```python
from build123d import *

# Parameters (mm, degrees)
SKETCH_1_W                     = 305.5
SKETCH_1_H                     = 1221.15
EXTRUDE_1_DEPTH                = 4.75
CUT_EXTRUDE_2_DEPTH            = 4.75
SPLIT_BODIES_1_SURFACE_1_BACK  = 1259.793
SPLIT_BODIES_1_SURFACE_1_DEPTH = 2519.586


with BuildPart() as part:
    # 草圖1 → 填料-伸長1 (new body)
    with BuildSketch(Plane.XY):
        Rectangle(SKETCH_1_W, SKETCH_1_H)
    extrude(amount=EXTRUDE_1_DEPTH)

    # 草圖2 → 除料-伸長2 (cut)
    with BuildSketch(Plane.XY.offset(4.75)):
        Polygon((100.025, 354.412698413), (100.025, 304.423280423), (-83.25542328, 382.984126984), (-99.975, 390.137566138), (-99.975, 440.126984127), (83.30542328, 361.566137566), align=None)
        Polygon((57.189021164, 380.021164021), (57.189021164, 440.126984127), (100.025, 440.126984127), (100.025, 361.566137566), align=None)
        Polygon((50.035582011, 106.53968254), (57.189021164, 106.53968254), (57.189021164, 120.846560847), (100.025, 120.846560847), (100.025, 84.994708995), (71.453571429, 56.55026455), (50.035582011, 56.55026455), align=None)
        Polygon((-71.403571429, 56.55026455), (-99.975, 84.994708995), (-99.975, 120.846560847), (-57.096693122, 120.846560847), (-57.096693122, 106.53968254), (-21.414153439, 106.53968254), (-21.414153439, 120.846560847), (21.464153439, 120.846560847), (21.464153439, 85.121693122), (-7.107275132, 56.55026455), align=None)
        Polygon((-21.414153439, 142.264550265), (-57.096693122, 142.264550265), (-57.096693122, 127.830687831), (-99.975, 128), (-99.975, 163.682539683), (-71.403571429, 192.423280423), (71.453571429, 192.253968254), (100.025, 163.682539683), (100.025, 127.830687831), (57.189021164, 127.830687831), (57.189021164, 142.264550265), (21.464153439, 142.264550265), (21.464153439, 128), (-21.414153439, 128), align=None)
        Polygon((21.591137566, -141.164021164), (57.189021164, -141.164021164), (57.189021164, -127.026455026), (100.025, -127.026455026), (100.025, -162.878306878), (71.453571429, -191.322751323), (7.157275132, -191.322751323), (0.046164021, -184.042328042), (-6.980291005, -191.44973545), (-71.276587302, -191.44973545), (-99.848015873, -163.047619048), (-99.975, -127.026455026), (-57.096693122, -127.026455026), (-56.969708995, -141.333333333), (-21.24484127, -141.333333333), (-21.414153439, -127.026455026), (21.29484127, -126.899470899), (21.29484127, -127.153439153), (21.591137566, -127.153439153), align=None)
        Polygon((50.035582011, -55.44973545), (71.453571429, -55.44973545), (100.025, -84.19047619), (100.025, -120.042328042), (57.189021164, -120.042328042), (57.189021164, -105.608465608), (50.035582011, -105.608465608), align=None)
        Polygon((-49.985582011, -105.608465608), (-57.096693122, -105.608465608), (-57.096693122, -120.042328042), (-99.975, -119.873015873), (-99.975, -84.19047619), (-71.403571429, -55.44973545), (-49.985582011, -55.44973545), align=None)
        Polygon((50.035582011, -389.206349206), (57.189021164, -389.206349206), (57.189021164, -374.899470899), (100.025, -374.899470899), (100.025, -410.751322751), (71.453571429, -439.195767196), (50.035582011, -439.195767196), align=None)
        Polygon((-71.403571429, -439.195767196), (-99.975, -410.751322751), (-99.975, -374.899470899), (-57.096693122, -374.899470899), (-57.096693122, -389.206349206), (-21.414153439, -389.206349206), (-21.414153439, -374.899470899), (21.464153439, -374.899470899), (21.464153439, -410.624338624), (-7.107275132, -439.195767196), align=None)
        Polygon((-21.414153439, -353.481481481), (-57.096693122, -353.481481481), (-57.096693122, -367.915343915), (-99.975, -367.746031746), (-99.975, -332.063492063), (-71.403571429, -303.322751323), (71.453571429, -303.492063492), (100.025, -332.063492063), (100.025, -367.915343915), (57.189021164, -367.915343915), (57.189021164, -353.481481481), (21.464153439, -353.481481481), (21.464153439, -367.746031746), (-21.414153439, -367.746031746), align=None)
    extrude(amount=-CUT_EXTRUDE_2_DEPTH, mode=Mode.SUBTRACT)

    # Split Bodies 1: cut with a surface, the side it looks to stays
    # Split Bodies 1 surface: a surface, the sketch's curves swept straight by 2519.586 mm
    with BuildLine(Plane.XY.offset(4.75).offset(-SPLIT_BODIES_1_SURFACE_1_BACK), mode=Mode.PRIVATE) as split_bodies_1_surface_1_path:
        Line((-152.75, 205.025), (152.75, 205.025))
    split_bodies_1_surface_1 = Shell.extrude(split_bodies_1_surface_1_path.wire(), (0 * SPLIT_BODIES_1_SURFACE_1_DEPTH, 0 * SPLIT_BODIES_1_SURFACE_1_DEPTH, 1 * SPLIT_BODIES_1_SURFACE_1_DEPTH))
    split(bisect_by=split_bodies_1_surface_1, keep=Keep.TOP)


solid = part.part
```
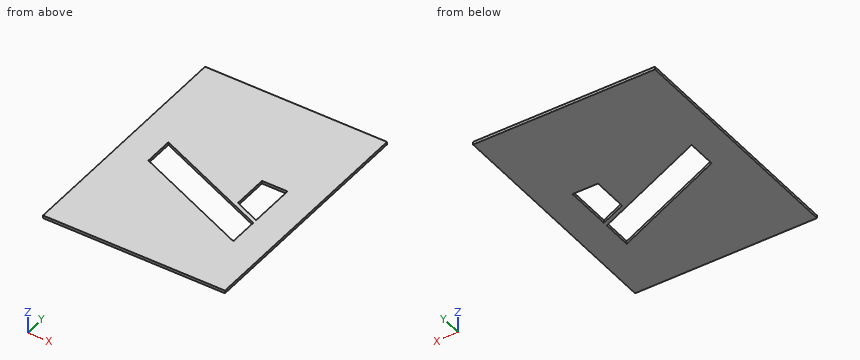
Design review of the part built by this model. Coordinates are the model's own, in mm. Round coordinates to 2 decimals unless told otherwise and drop trailing zeros. Write each loop counter-clockwise with the first axis right and the second up, starting at its lowest first coordinate (ties: lowest second). Pieces come first, ordered by that corner, then holes. Notation, with made-up numbers: (18, 0.5) -> (46, 0.5) arc R20 ccw to (46, 20.5) -> close; hole circle Ø4 at (57.25, 50.25). An arc over 180 degrees is marked (long way). Answer in a Markdown table with one row per item.
Q1. Take a section at B-B, the plane x = 33. State the section outline as (y, z) points (3 decimals), then the cut area to 3 significant figures.
The answers:
| item | result |
|---|---|
| outline | (205.025, 0) -> (333.153, 0) -> (333.153, 4.75) -> (205.025, 4.75) -> close; (383.129, 0) -> (610.575, 0) -> (610.575, 4.75) -> (383.129, 4.75) -> close |
| area | 1,690 mm² |
Q2. Take a section at C-C, the plane y = 402. State the section outline as (x, z) points (3 decimals), then the cut area to 3 significant figures.
The answers:
| item | result |
|---|---|
| outline | (-152.75, 0) -> (-99.975, 0) -> (-99.975, 4.75) -> (-152.75, 4.75) -> close; (-11.026, 0) -> (57.189, 0) -> (57.189, 4.75) -> (-11.026, 4.75) -> close; (100.025, 0) -> (152.75, 0) -> (152.75, 4.75) -> (100.025, 4.75) -> close |
| area | 825 mm² |
Q3. Take a section at A-A, the plane z = 1. State the section outline as (x, y) points (3 decimals).
The answers:
| item | result |
|---|---|
| outline | (-152.75, 205.025) -> (152.75, 205.025) -> (152.75, 610.575) -> (-152.75, 610.575) -> close; hole (-99.975, 390.138) -> (-83.255, 382.984) -> (100.025, 304.423) -> (100.025, 354.413) -> (83.305, 361.566) -> (-99.975, 440.127) -> close; hole (57.189, 380.021) -> (100.025, 361.566) -> (100.025, 440.127) -> (57.189, 440.127) -> close |
Q4. Take a section at D-D, the plane y = 319.5. State the section outline as (x, z) points (3 decimals).
The answers:
| item | result |
|---|---|
| outline | (-152.75, 0) -> (64.851, 0) -> (64.851, 4.75) -> (-152.75, 4.75) -> close; (100.025, 0) -> (152.75, 0) -> (152.75, 4.75) -> (100.025, 4.75) -> close |
Q5. To check wall thickness, follow L1, parallel to X at y = 434.5, z = 0.7 (3 decimals); L2, parallel to X at y = 382, z = 2.25 (3 decimals); L3, parallel to Y at x = -89.5, z = 3.35 (3 decimals). State the ranges of each line that lie inside material, in increasing order. Write a range as [from, to].
The answers:
| item | result |
|---|---|
| L1 | [-152.75, -99.975], [-86.847, 57.189], [100.025, 152.75] |
| L2 | [-152.75, -80.959], [35.634, 57.189], [100.025, 152.75] |
| L3 | [205.025, 385.656], [435.637, 610.575] |
